Read the model definition and answer for the solid it produces. Units are mm, in the model's axes. Face numbers are marked on the shaded views. Coordinates: 2 decimals unless noted, no trailing zeros. One line per item, written item: value. Start each with the question number.
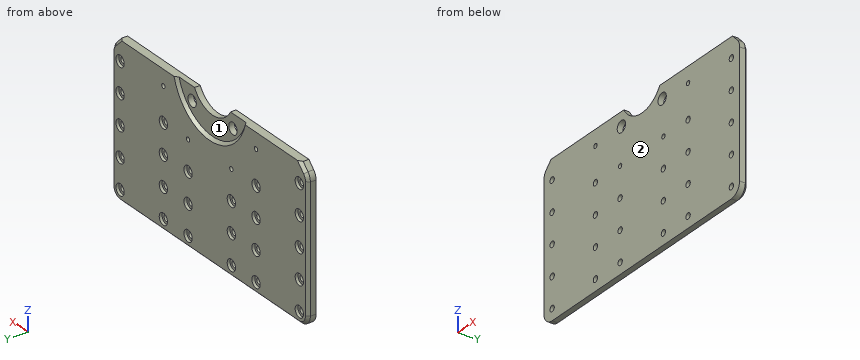
from build123d import *

# Parameters (mm, degrees)
EXTRUDE_1_DEPTH               = 3
HOLE_WIZARD_M2_1_AT_2_COUNT   = 2
HOLE_WIZARD_M2_1_AT_2_PITCH   = 21
PATTERN_LINEAR_1_COUNT        = 3
PATTERN_LINEAR_1_PITCH        = 33
PATTERN_LINEAR_2_COUNT        = 3
PATTERN_LINEAR_2_PITCH        = 10.5
PATTERN_LINEAR_3_COUNT        = 2
PATTERN_LINEAR_3_PITCH        = 31.5
HOLE_WIZARD_M2_1_2_AT_2_COUNT = 2
HOLE_WIZARD_M2_1_2_AT_2_PITCH = 16.970562748
SKETCH_8_R                    = 17
CUT_EXTRUDE_1_DEPTH           = 1
SKETCH_9_R                    = 2.025
CUT_EXTRUDE_2_DEPTH           = 75.994999833
PATTERN_CIRCULAR_1_COUNT      = 2
PATTERN_CIRCULAR_1_ANGLE      = 90
FILLET_1_R                    = 4
CHAMFER_1_SIZE                = 1
SKETCH_11_W                   = 95
SKETCH_11_H                   = 10
CUT_EXTRUDE_3_DEPTH           = 76.028327984


with BuildPart() as part:
    # ｽｹｯﾁ1 → ﾎﾞｽ - 押し出し1 (new body)
    with BuildSketch(Plane(origin=(0, 0, 0), x_dir=(1, 0, 0), z_dir=(0, 1, 0))):
        with BuildLine():
            Line((-10.05, 0), (-39, 0))
            Line((-39, 0), (-47.5, 8.5))
            Line((-47.5, 8.5), (-47.5, 58))
            Line((-47.5, 58), (47.5, 58))
            Line((47.5, 58), (47.5, 8.5))
            Line((47.5, 8.5), (39, 0))
            Line((39, 0), (10.05, 0))
            ThreePointArc((10.05, 0), (0, 10.05), (-10.05, 0))
        make_face()
    extrude(amount=EXTRUDE_1_DEPTH)

    # ｽｹｯﾁ3 → Hole Wizard M2 _1 (revolve, cut)
    with BuildSketch(Plane(origin=(-43.5, 3, -54), x_dir=(0, 0, 1), z_dir=(1, 0, 0))):
        Polygon((0, 0), (0, 4.63090365), (1.05, 4), (1.05, 1), (2, 1), (2, 0), align=None)
    hole_wizard_m2_1 = revolve(axis=Axis((-43.5, 9.35, -54), (0, -1, 0)), mode=Mode.SUBTRACT)

    # Hole Wizard M2 _1 at 2: Hole Wizard M2 _1 ×2
    with Locations(*[(i * HOLE_WIZARD_M2_1_AT_2_PITCH, 0, 0) for i in range(1, HOLE_WIZARD_M2_1_AT_2_COUNT)]):
        add(hole_wizard_m2_1, mode=Mode.SUBTRACT)

    # 直線ﾊﾟﾀｰﾝ1: Hole Wizard M2 _1 ×3
    with Locations(*[(i * PATTERN_LINEAR_1_PITCH, 0, 0) for i in range(1, PATTERN_LINEAR_1_COUNT)]):
        add(hole_wizard_m2_1, mode=Mode.SUBTRACT)

    # 直線ﾊﾟﾀｰﾝ1 copy 1 sketch → 直線ﾊﾟﾀｰﾝ1 copy 1 (revolve, cut)
    with BuildSketch(Plane(origin=(10.5, 3, -54), x_dir=(0, 0, 1), z_dir=(1, 0, 0))):
        Polygon((0, 0), (0, 4.63090365), (1.05, 4), (1.05, 1), (2, 1), (2, 0), align=None)
    revolve(axis=Axis((10.5, 9.35, -54), (0, -1, 0)), mode=Mode.SUBTRACT)

    # 直線ﾊﾟﾀｰﾝ1 copy 2 sketch → 直線ﾊﾟﾀｰﾝ1 copy 2 (revolve, cut)
    with BuildSketch(Plane(origin=(43.5, 3, -54), x_dir=(0, 0, 1), z_dir=(1, 0, 0))):
        Polygon((0, 0), (0, 4.63090365), (1.05, 4), (1.05, 1), (2, 1), (2, 0), align=None)
    revolve(axis=Axis((43.5, 9.35, -54), (0, -1, 0)), mode=Mode.SUBTRACT)

    # 直線ﾊﾟﾀｰﾝ2: Hole Wizard M2 _1 ×3
    with Locations(*[(0, 0, i * PATTERN_LINEAR_2_PITCH) for i in range(1, PATTERN_LINEAR_2_COUNT)]):
        add(hole_wizard_m2_1, mode=Mode.SUBTRACT)

    # 直線ﾊﾟﾀｰﾝ2 copy 1 sketch → 直線ﾊﾟﾀｰﾝ2 copy 1 (revolve, cut)
    with BuildSketch(Plane(origin=(-22.5, 3, -43.5), x_dir=(0, 0, 1), z_dir=(1, 0, 0))):
        Polygon((0, 0), (0, 4.63090365), (1.05, 4), (1.05, 1), (2, 1), (2, 0), align=None)
    revolve(axis=Axis((-22.5, 9.35, -43.5), (0, -1, 0)), mode=Mode.SUBTRACT)

    # 直線ﾊﾟﾀｰﾝ2 copy 2 sketch → 直線ﾊﾟﾀｰﾝ2 copy 2 (revolve, cut)
    with BuildSketch(Plane(origin=(-22.5, 3, -33), x_dir=(0, 0, 1), z_dir=(1, 0, 0))):
        Polygon((0, 0), (0, 4.63090365), (1.05, 4), (1.05, 1), (2, 1), (2, 0), align=None)
    revolve(axis=Axis((-22.5, 9.35, -33), (0, -1, 0)), mode=Mode.SUBTRACT)

    # 直線ﾊﾟﾀｰﾝ2 copy 3 sketch → 直線ﾊﾟﾀｰﾝ2 copy 3 (revolve, cut)
    with BuildSketch(Plane(origin=(-10.5, 3, -43.5), x_dir=(0, 0, 1), z_dir=(1, 0, 0))):
        Polygon((0, 0), (0, 4.63090365), (1.05, 4), (1.05, 1), (2, 1), (2, 0), align=None)
    revolve(axis=Axis((-10.5, 9.35, -43.5), (0, -1, 0)), mode=Mode.SUBTRACT)

    # 直線ﾊﾟﾀｰﾝ2 copy 4 sketch → 直線ﾊﾟﾀｰﾝ2 copy 4 (revolve, cut)
    with BuildSketch(Plane(origin=(-10.5, 3, -33), x_dir=(0, 0, 1), z_dir=(1, 0, 0))):
        Polygon((0, 0), (0, 4.63090365), (1.05, 4), (1.05, 1), (2, 1), (2, 0), align=None)
    revolve(axis=Axis((-10.5, 9.35, -33), (0, -1, 0)), mode=Mode.SUBTRACT)

    # 直線ﾊﾟﾀｰﾝ2 copy 5 sketch → 直線ﾊﾟﾀｰﾝ2 copy 5 (revolve, cut)
    with BuildSketch(Plane(origin=(22.5, 3, -43.5), x_dir=(0, 0, 1), z_dir=(1, 0, 0))):
        Polygon((0, 0), (0, 4.63090365), (1.05, 4), (1.05, 1), (2, 1), (2, 0), align=None)
    revolve(axis=Axis((22.5, 9.35, -43.5), (0, -1, 0)), mode=Mode.SUBTRACT)

    # 直線ﾊﾟﾀｰﾝ2 copy 6 sketch → 直線ﾊﾟﾀｰﾝ2 copy 6 (revolve, cut)
    with BuildSketch(Plane(origin=(22.5, 3, -33), x_dir=(0, 0, 1), z_dir=(1, 0, 0))):
        Polygon((0, 0), (0, 4.63090365), (1.05, 4), (1.05, 1), (2, 1), (2, 0), align=None)
    revolve(axis=Axis((22.5, 9.35, -33), (0, -1, 0)), mode=Mode.SUBTRACT)

    # 直線ﾊﾟﾀｰﾝ2 copy 7 sketch → 直線ﾊﾟﾀｰﾝ2 copy 7 (revolve, cut)
    with BuildSketch(Plane(origin=(10.5, 3, -43.5), x_dir=(0, 0, 1), z_dir=(1, 0, 0))):
        Polygon((0, 0), (0, 4.63090365), (1.05, 4), (1.05, 1), (2, 1), (2, 0), align=None)
    revolve(axis=Axis((10.5, 9.35, -43.5), (0, -1, 0)), mode=Mode.SUBTRACT)

    # 直線ﾊﾟﾀｰﾝ2 copy 8 sketch → 直線ﾊﾟﾀｰﾝ2 copy 8 (revolve, cut)
    with BuildSketch(Plane(origin=(10.5, 3, -33), x_dir=(0, 0, 1), z_dir=(1, 0, 0))):
        Polygon((0, 0), (0, 4.63090365), (1.05, 4), (1.05, 1), (2, 1), (2, 0), align=None)
    revolve(axis=Axis((10.5, 9.35, -33), (0, -1, 0)), mode=Mode.SUBTRACT)

    # 直線ﾊﾟﾀｰﾝ2 copy 9 sketch → 直線ﾊﾟﾀｰﾝ2 copy 9 (revolve, cut)
    with BuildSketch(Plane(origin=(43.5, 3, -43.5), x_dir=(0, 0, 1), z_dir=(1, 0, 0))):
        Polygon((0, 0), (0, 4.63090365), (1.05, 4), (1.05, 1), (2, 1), (2, 0), align=None)
    revolve(axis=Axis((43.5, 9.35, -43.5), (0, -1, 0)), mode=Mode.SUBTRACT)

    # 直線ﾊﾟﾀｰﾝ2 copy 10 sketch → 直線ﾊﾟﾀｰﾝ2 copy 10 (revolve, cut)
    with BuildSketch(Plane(origin=(43.5, 3, -33), x_dir=(0, 0, 1), z_dir=(1, 0, 0))):
        Polygon((0, 0), (0, 4.63090365), (1.05, 4), (1.05, 1), (2, 1), (2, 0), align=None)
    revolve(axis=Axis((43.5, 9.35, -33), (0, -1, 0)), mode=Mode.SUBTRACT)

    # 直線ﾊﾟﾀｰﾝ3: Hole Wizard M2 _1 ×2
    with Locations(*[(0, 0, i * PATTERN_LINEAR_3_PITCH) for i in range(1, PATTERN_LINEAR_3_COUNT)]):
        add(hole_wizard_m2_1, mode=Mode.SUBTRACT)

    # 直線ﾊﾟﾀｰﾝ3 copy 1 sketch → 直線ﾊﾟﾀｰﾝ3 copy 1 (revolve, cut)
    with BuildSketch(Plane(origin=(-22.5, 3, -22.5), x_dir=(0, 0, 1), z_dir=(1, 0, 0))):
        Polygon((0, 0), (0, 4.63090365), (1.05, 4), (1.05, 1), (2, 1), (2, 0), align=None)
    revolve(axis=Axis((-22.5, 9.35, -22.5), (0, -1, 0)), mode=Mode.SUBTRACT)

    # ｽｹｯﾁ5 → Hole Wizard M2 _1 2 (revolve, cut)
    with BuildSketch(Plane(origin=(-10.5, 3, -22.5), x_dir=(0, 0, 1), z_dir=(1, 0, 0))):
        Polygon((0, 0), (0, 6.480688495), (0.8, 6), (0.8, 0), align=None)
    hole_wizard_m2_1_2 = revolve(axis=Axis((-10.5, 9.35, -22.5), (0, -1, 0)), mode=Mode.SUBTRACT)

    # Hole Wizard M2 _1 2 at 2: Hole Wizard M2 _1 2 ×2
    with Locations(*[Vector(-0.7071067811865469, 0, 0.7071067811865482) * (i * HOLE_WIZARD_M2_1_2_AT_2_PITCH) for i in range(1, HOLE_WIZARD_M2_1_2_AT_2_COUNT)]):
        add(hole_wizard_m2_1_2, mode=Mode.SUBTRACT)

    # ｽｹｯﾁ7 → M2 なべ頭ねじ用座ぐり穴2 (revolve, cut)
    with BuildSketch(Plane(origin=(-43.5, 3, -12), x_dir=(0, 0, 1), z_dir=(1, 0, 0))):
        Polygon((0, 0), (0, 6.63090365), (1.05, 6), (1.05, 1), (2, 1), (2, 0), align=None)
    hole_wizard_m2_2 = revolve(axis=Axis((-43.5, 9.35, -12), (0, -1, 0)), mode=Mode.SUBTRACT)

    # ﾐﾗｰ1: Hole Wizard M2 _1 2, M2 なべ頭ねじ用座ぐり穴2 across plane
    add(hole_wizard_m2_1_2.mirror(Plane(origin=(0, 0, 0), x_dir=(0, 0, 1), z_dir=(1, 0, 0))), mode=Mode.SUBTRACT)
    add(hole_wizard_m2_2.mirror(Plane(origin=(0, 0, 0), x_dir=(0, 0, 1), z_dir=(1, 0, 0))), mode=Mode.SUBTRACT)

    # ﾐﾗｰ1 copy 1 sketch → ﾐﾗｰ1 copy 1 (revolve, cut)
    with BuildSketch(Plane(origin=(43.5, 3, -22.5), x_dir=(0, 0, 1), z_dir=(-1, 0, 0))):
        Polygon((0, 0), (0, -4.63090365), (1.05, -4), (1.05, -1), (2, -1), (2, 0), align=None)
    revolve(axis=Axis((43.5, 9.35, -22.5), (0, 1, 0)), mode=Mode.SUBTRACT)

    # ﾐﾗｰ1 copy 2 sketch → ﾐﾗｰ1 copy 2 (revolve, cut)
    with BuildSketch(Plane(origin=(22.5, 3, -22.5), x_dir=(0, 0, 1), z_dir=(-1, 0, 0))):
        Polygon((0, 0), (0, -4.63090365), (1.05, -4), (1.05, -1), (2, -1), (2, 0), align=None)
    revolve(axis=Axis((22.5, 9.35, -22.5), (0, 1, 0)), mode=Mode.SUBTRACT)

    # ﾐﾗｰ1 copy 3 sketch → ﾐﾗｰ1 copy 3 (revolve, cut)
    with BuildSketch(Plane(origin=(43.5, 3, -54), x_dir=(0, 0, 1), z_dir=(-1, 0, 0))):
        Polygon((0, 0), (0, -4.63090365), (1.05, -4), (1.05, -1), (2, -1), (2, 0), align=None)
    revolve(axis=Axis((43.5, 9.35, -54), (0, 1, 0)), mode=Mode.SUBTRACT)

    # ﾐﾗｰ1 copy 4 sketch → ﾐﾗｰ1 copy 4 (revolve, cut)
    with BuildSketch(Plane(origin=(22.5, 3, -54), x_dir=(0, 0, 1), z_dir=(-1, 0, 0))):
        Polygon((0, 0), (0, -4.63090365), (1.05, -4), (1.05, -1), (2, -1), (2, 0), align=None)
    revolve(axis=Axis((22.5, 9.35, -54), (0, 1, 0)), mode=Mode.SUBTRACT)

    # ﾐﾗｰ1 copy 5 sketch → ﾐﾗｰ1 copy 5 (revolve, cut)
    with BuildSketch(Plane(origin=(22.5, 3, -10.5), x_dir=(0, 0, 1), z_dir=(-1, 0, 0))):
        Polygon((0, 0), (0, -6.480688495), (0.8, -6), (0.8, 0), align=None)
    revolve(axis=Axis((22.5, 9.35, -10.5), (0, 1, 0)), mode=Mode.SUBTRACT)

    # ｽｹｯﾁ8 → ｶｯﾄ - 押し出し1 (cut)
    with BuildSketch(Plane(origin=(0, 3, 0), x_dir=(1, 0, 0), z_dir=(0, 1, 0))):
        Circle(SKETCH_8_R)
    extrude(amount=-CUT_EXTRUDE_1_DEPTH, mode=Mode.SUBTRACT)

    # ｽｹｯﾁ9 → ｶｯﾄ - 押し出し2 (cut, through all)
    with BuildSketch(Plane(origin=(0, 2, 0), x_dir=(1, 0, 0), z_dir=(0, 1, 0))):
        with Locations(Location((-9.899494937, 9.899494937, 0), (0, 0, 270))):
            Circle(SKETCH_9_R)
    cut_extrude_2 = extrude(amount=-CUT_EXTRUDE_2_DEPTH, mode=Mode.SUBTRACT)

    # 円形ﾊﾟﾀｰﾝ1: ｶｯﾄ - 押し出し2 ×2 about axis
    pattern_circular_1_axis = Axis((0, 3, 0), (0, -1, 0))
    for i in range(1, PATTERN_CIRCULAR_1_COUNT):
        add(cut_extrude_2.rotate(pattern_circular_1_axis, i * PATTERN_CIRCULAR_1_ANGLE / (PATTERN_CIRCULAR_1_COUNT - 1)), mode=Mode.SUBTRACT)

    # ﾌｨﾚｯﾄ1
    fillet_1_edges = [part.edges().sort_by_distance(p)[0] for p in [
        (-47.5, 1.5, -8.5),
        (-47.5, 1.5, -58),
        (47.5, 1.5, -58),
        (47.5, 1.5, -8.5),
        (39, 1.5, 0),
        (-39, 1.5, 0),
    ]]
    fillet(fillet_1_edges, radius=FILLET_1_R)

    # 面取り1
    chamfer_1_edges = [part.edges().sort_by_distance(p)[0] for p in [
        (0, 3, -17),
        (27.171572875, 3, 0),
        (38.87387948, 3, -0.30448187),
        (43.25, 3, -4.25),
        (47.19551813, 3, -8.62612052),
        (47.5, 3, -32.078427125),
        (-27.171572875, 3, 0),
        (46.328427125, 3, -56.828427125),
        (-38.87387948, 3, -0.30448187),
        (0, 3, -58),
        (-43.25, 3, -4.25),
        (-46.328427125, 3, -56.828427125),
        (-47.19551813, 3, -8.62612052),
        (-47.5, 3, -32.078427125),
    ]]
    chamfer(chamfer_1_edges, length=CHAMFER_1_SIZE - 0.0001)  # a hair under: the kernel refuses the full size

    # ｽｹｯﾁ11 → ｶｯﾄ - 押し出し3 (cut, through all)
    with BuildSketch(Plane(origin=(0, 3, 0), x_dir=(1, 0, 0), z_dir=(0, 1, 0))):
        Rectangle(SKETCH_11_W, SKETCH_11_H)
    extrude(amount=-CUT_EXTRUDE_3_DEPTH, mode=Mode.SUBTRACT)


solid = part.part
1) Determine the mould class of the marked faces 1 and 2 for opening direction X: released by +X, released by -X, zero draft, split by the parting line, or undercut.
2) Straight lines are drawn through the part: L1, parallel to Z at x = 43, y = 0.85; L2, parallel to Z at x = -10.5, y = 1.3; L3, parallel to X at y = 2.5, z = -12. For each, find the intervals that lie inside material, in ascending order.
3) Section A-A, the plane z = -33 is taken. State how many separate pieces and enclosed holes the cut face has, and give its area (3 significant figures).
4) A flat-ended cylindrical pin translates along its axis: P1, Ø2.5, axis at x = 22.5, z = -22.5, coming from the +Y side. Find the tip coordinate at first contact, or state that the pin passes through.
Answer below:
1. face 1: undercut
1. face 2: zero draft
2. L1: -58 to -54.92, -53.08 to -44.42, -42.58 to -33.92, -32.08 to -23.42, -21.58 to -12.92, -11.08 to -5
2. L2: -58 to -55.05, -52.95 to -44.55, -42.45 to -34.05, -31.95 to -23.3, -21.7 to -11.83, -7.97 to -5
2. L3: -47 to -45.5, -41.5 to -12.74, 12.74 to 41.5, 45.5 to 47
3. separate pieces: 7
3. enclosed holes: 0
3. area: 235 mm2
4. P1: y = 2
